Model file for the job. Use its own axes, mm. Face numbers are marked on the shaded views. A direction names the side the tool comes from. Coordinates: 2 decimals unless noted, no trailing zeros. Write each loop counter-clockwise with the first axis right and the second up, starting at its lowest first coordinate (ties: lowest second). Pieces come first, ordered by that corner, then holes. Notation, with made-up numbers: M 76,34.25 L 119,34.25 A11 ccw 119,55.25 Z; hole C 81.25,18.5 d5. An arc over 180 degrees is marked long. Put each result on its own line as item: value. Start each with the question number.
Q1. Cut at C-C (y = 30). Write the cut outline in (x, z).
Q2. Pull direction X, two halves, no side cores. Call the marked faces 1, 2, 3 and 4: pulls with the +X half, pulls with the -X half, needs draft (parallel to the pull), parting line crosses it, or undercut.
Q3. Which spindle directions (+Z, -Z, +X, -X, +Y, -Y) get a long thin tool onto all of the face, cutting with end or side? Do the marked faces 5, 6 and 7. Say none if no direction does.
Q4. Drop flat-ended pins along their axis: pin 1 (10 mm diameter, centred on x = 47, y = 13, fed in from +Z); pin 2 (6 mm diameter, centred on y = 20, z = 14, fed in from +X); pin 3 (2 mm diameter, centred on x = -29.5, z = 15.5, fed in from +Y); pin 4 (3 mm diameter, centred on y = 16, z = 8.5, fed in from -X). Give the stop position or say it passes through.
Q5. Drill centre lines: line 1 along X through (y, z) = (22, 9); line 2 along Y through (x, z) = (-12.5, 11); line 3 along X through (y, z) = (15.5, 24). Where is each one in solid material? Low to high.
Q6. Cut at B-B (x = -23). Write the cut outline in (y, z).
Q7. Cut at D-D (x = 7). Write the cut outline in (y, z).
Q8. Cut at A-A (z = 8). Write the cut outline in (x, y), then the cut area to 3 significant figures.
```python
from build123d import *

# Parameters (mm, degrees)
F0_W     = 127.210148
F0_H     = 38.565968
F1_DEPTH = 5.08
F2_W     = 122.317444
F2_H     = 33.961081
F2_R     = 11.576806
F2_R_2   = 11.574122
F3_DEPTH = 25.4
F4_W     = 40.869429
F4_H     = 29.961394
F5_DEPTH = 22.86
F6_W     = 43.170862
F6_H     = 25.614712
F7_DEPTH = 20.32


with BuildPart() as f1:
    # F0 (on Top) → F1 (new body)
    with BuildSketch(Plane.XY):
        with Locations((4e-06, 22.161042)):
            Rectangle(F0_W, F0_H)
    extrude(amount=-F1_DEPTH)

    # F2 (on face) → F3 (join)
    with BuildSketch(Plane.XY):
        with Locations((-0.143906, 22.161044)):
            Rectangle(F2_W, F2_H)
        with Locations((-41.156225, 22.161044)):
            Circle(F2_R, mode=Mode.SUBTRACT)
        with Locations((42.16354, 22.161044)):
            Circle(F2_R_2, mode=Mode.SUBTRACT)
    extrude(amount=F3_DEPTH)

    # F4 (on face) → F5 (join)
    with BuildSketch(Plane.XY.offset(25.4)):
        with Locations((0.288312, 22.15811)):
            Rectangle(F4_W, F4_H)
    extrude(amount=-F5_DEPTH)

    # F6 (on face) → F7 (cut)
    with BuildSketch(Plane.XY.offset(25.4)):
        with Locations((1.151221, 23.456169)):
            Rectangle(F6_W, F6_H)
    extrude(amount=-F7_DEPTH, mode=Mode.SUBTRACT)


solid = f1.part
```
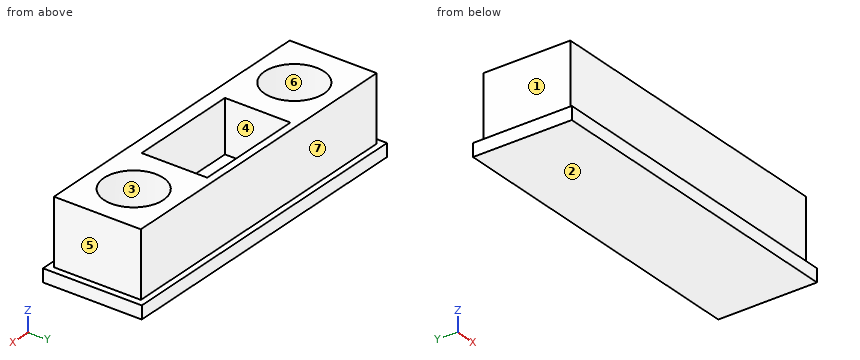
Computed values:
1. outline: M -63.61,-5.08 L 63.61,-5.08 L 63.61,0 L 61.01,0 L 61.01,25.4 L 50.68,25.4 L 50.68,0 L 33.65,0 L 33.65,25.4 L 22.74,25.4 L 22.74,5.08 L -20.43,5.08 L -20.43,25.4 L -32.64,25.4 L -32.64,0 L -49.68,0 L -49.68,25.4 L -61.3,25.4 L -61.3,0 L -63.61,0 Z
2. face 1: pulls with the -X half
2. face 2: needs draft
2. face 3: undercut
2. face 4: undercut
3. face 5: +Z, +X, +Y, -Y
3. face 6: +Z
3. face 7: +Z, +X, -X, +Y
4. pin 1: z = 25.4
4. pin 2: x = 61.01
4. pin 3: y = 39.14
4. pin 4: x = -61.3
5. line 1: -61.3 to -52.73, -29.58 to -20.43, 22.74 to 30.59, 53.74 to 61.01
5. line 2: 5.18 to 10.65, 36.26 to 39.14
5. line 3: -61.3 to -50.62, -31.69 to -20.43, 22.74 to 32.7, 51.63 to 61.01
6. outline: M 2.88,-5.08 L 41.44,-5.08 L 41.44,0 L 39.14,0 L 39.14,25.4 L 5.18,25.4 L 5.18,0 L 2.88,0 Z
7. outline: M 2.88,-5.08 L 41.44,-5.08 L 41.44,0 L 39.14,0 L 39.14,25.4 L 36.26,25.4 L 36.26,5.08 L 10.65,5.08 L 10.65,25.4 L 5.18,25.4 L 5.18,0 L 2.88,0 Z
8. outline: M -61.3,5.18 L 61.01,5.18 L 61.01,39.14 L -61.3,39.14 Z; hole C -41.16,22.16 d23.15; hole M -20.43,10.65 L 22.74,10.65 L 22.74,36.26 L -20.43,36.26 Z; hole C 42.16,22.16 d23.15
8. area: 2,210 mm2
